Can you work these out from the model? Positions are in its coordinate system, mm. Face numbers are marked on the shaded views. A direction names the side the tool comes from. Give positions to 0.01 mm unless a question says otherwise; leave off trailing zeros. Write each loop counter-clockwise with the first axis right and the second up, starting at its lowest first coordinate (ties: lowest second). Pieces come first, ordered by that corner, then holes.
Autodesk Inventor part; units mm, degrees
ref_plane "YZ Plane" through (0, 0, 0) normal (1, 0, 0) x (0, 1, 0)
ref_plane "XZ Plane" through (0, 0, 0) normal (0, 1, 0) x (-1, 0, 0)
ref_plane "XY Plane" through (0, 0, 0) normal (0, 0, 1) x (1, 0, 0)
sketch "スケッチ1" plane through (0, 0, 0) normal (0, 0, 1) x (1, 0, 0)
  circle A0 centre (0, 0) radius 46.9412
  dimension "d3" = 93.8824
extrude "押し出し1" add sketch "スケッチ1" along normal blind 10.5
sketch "スケッチ2" plane through (0, 0, 10.5) normal (0, 0, 1) x (1, 0, 0)
  circle A0 centre (0, 0) radius 46.9412
  arc A1 (35.7361, 3.8892) -> (3.8892, 35.7361) centre (0, 0) ccw
  circle A2 centre (29.2617, 29.2617) radius 2.1
  circle A3 centre (-39.9723, 10.7105) radius 2.1
  circle A4 centre (10.7105, -39.9723) radius 2.1
  circle A5 centre (0, 0) radius 35.9471
  dimension "d4" = 4.2
extrude "押し出し2" cut sketch "スケッチ2" against normal blind 5 contours A5 A1
sketch "スケッチ3" plane through (0, 0, 10.5) normal (0, 0, 1) x (1, 0, 0)
  circle A0 centre (0, 0) radius 46.9412
  arc A1 (-5.0225, 35.5945) -> (35.5945, -5.0225) centre (0, 0) ccw
  arc A2 (35.7361, 3.8892) -> (3.8892, 35.7361) centre (0, 0) ccw
  circle A3 centre (29.2617, 29.2617) radius 2.1
  circle A4 centre (-39.9723, 10.7105) radius 2.1
  circle A5 centre (10.7105, -39.9723) radius 2.1
  circle A6 centre (0, 0) radius 35.9471
  dimension "d7" = 4.2
extrude "押し出し3" cut sketch "スケッチ3" against normal blind 10.5 contours A3 | A4 | A5
sketch "スケッチ4" plane through (0, 0, 5.5) normal (0, 0, 1) x (1, 0, 0)
  circle A0 centre (0, 0) radius 10.5
  circle A1 centre (0, 0) radius 10.5
extrude "押し出し4" cut sketch "スケッチ4" against normal blind 10.5
sketch "スケッチ5" plane through (0, 0, 5.5) normal (0, 0, 1) x (1, 0, 0)
  circle A0 centre (0, 0) radius 10.5
  circle A1 centre (0, 0) radius 35.9471
  circle A2 centre (0, 0) radius 13.5
  circle A3 centre (0, 0) radius 32.9471
  dimension "d12" = 3
  dimension "d13" = 3
extrude "押し出し5" cut sketch "スケッチ5" against normal blind 2 contours A3
sketch "スケッチ6" plane through (0, 0, 5.5) normal (0, 0, 1) x (1, 0, 0)
  point P0 (0, 0)
sketch "スケッチ7" plane through (0, 0, 5.5) normal (0, 0, 1) x (1, 0, 0)
  circle A0 centre (0, 0) radius 38.9471
  circle A1 centre (0, 0) radius 35.9471
  dimension "d16" = 3
extrude "押し出し6" cut sketch "スケッチ7" along normal blind 2.5
properties part number "fix_plate_2"
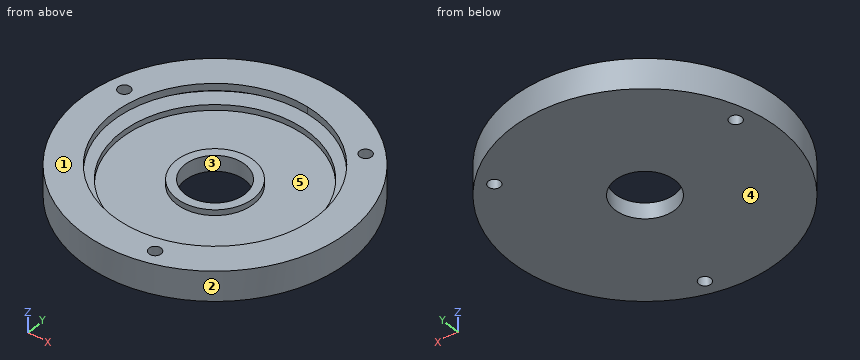
(1) Imagine slicing it at C-C, the plane z = 2. Write out the boundary of the cut face in (x, y), plus the area to 3 significant figures.
Returned:
outline: circle Ø93.88 at (0, 0); hole circle Ø4.2 at (-39.97, 10.71); hole circle Ø21 at (0, 0); hole circle Ø4.2 at (10.71, -39.97); hole circle Ø4.2 at (29.26, 29.26)
area: 6,530 mm2
(2) Imagine slicing it at D-D, the plane y = 22.5. Write out the boundary of the cut face in (x, z).
Returned:
outline: (-41.2, 0) - (41.2, 0) - (41.2, 10.5) - (28.03, 10.5) - (28.03, 8) - (31.79, 8) - (31.79, 5.5) - (24.07, 5.5) - (24.07, 3.5) - (-24.07, 3.5) - (-24.07, 5.5) - (-31.79, 5.5) - (-31.79, 8) - (-28.03, 8) - (-28.03, 10.5) - (-41.2, 10.5) - close
(3) Imagine slicing it at B-B, the plane x = 1. Write out the boundary of the cut face in (y, z).
Returned:
outline: (-46.93, 0) - (-10.45, 0) - (-10.45, 5.5) - (-13.46, 5.5) - (-13.46, 3.5) - (-32.93, 3.5) - (-32.93, 5.5) - (-38.93, 5.5) - (-38.93, 8) - (-35.93, 8) - (-35.93, 10.5) - (-46.93, 10.5) - close; (10.45, 0) - (46.93, 0) - (46.93, 10.5) - (35.93, 10.5) - (35.93, 8) - (38.93, 8) - (38.93, 5.5) - (32.93, 5.5) - (32.93, 3.5) - (13.46, 3.5) - (13.46, 5.5) - (10.45, 5.5) - close
(4) Will these pins go through, and if not, where does the flat tip stop? P1, Ø23.5, axis at x = 2.5, y = -13, coming from the -Z side; P2, Ø5, axis at x = -27, y = -1, coming from the +Z side; P3, Ø4, axis at x = -12.5, z = 4, coming from the -Y side; P4, Ø13.5, axis at x = 6.5, y = -1, coming from the +Z side.
Returned:
P1: stops at z = 0
P2: stops at z = 3.5
P3: stops at y = -45.75
P4: stops at z = 5.5
(5) If I drill on L1, parallel to Y at x = 0, z = 4.45; L2, parallel to X at y = -11.5, z = 4.75; L3, parallel to Z at x = -10.5, y = -35, over which ranges is the centre line in solid material (lowest first)?
Returned:
L1: y = -46.94 to -32.95, -13.5 to -10.5, 10.5 to 13.5, 32.95 to 46.94
L2: x = -45.51 to -30.87, -7.07 to 7.07, 30.87 to 45.51
L3: z = 0 to 5.5, 8 to 10.5
(6) Imagine slicing it at A-A, the plane y = 0. Write out the boundary of the cut face in (x, z), plus the area to 3 significant figures.
Returned:
outline: (-46.94, 0) - (-10.5, 0) - (-10.5, 5.5) - (-13.5, 5.5) - (-13.5, 3.5) - (-32.95, 3.5) - (-32.95, 5.5) - (-38.95, 5.5) - (-38.95, 8) - (-35.95, 8) - (-35.95, 10.5) - (-46.94, 10.5) - close; (10.5, 0) - (46.94, 0) - (46.94, 10.5) - (35.95, 10.5) - (35.95, 8) - (38.95, 8) - (38.95, 5.5) - (32.95, 5.5) - (32.95, 3.5) - (13.5, 3.5) - (13.5, 5.5) - (10.5, 5.5) - close
area: 418 mm2
(7) If we mould it in two halves opening along X, with no side actions, what happens to the marked faces 1, 2 and 3? For each: +X half, -X half, draft (parallel to the pull), parting line (faces both ways), or undercut.
Returned:
face 1: draft
face 2: parting line
face 3: undercut
(8) For the marked faces 4 and 5, which set-ups out of +Z, -Z, +X, -X, +Y, -Y let a thin tool reach every point of the face, with its end or its side?
Returned:
face 4: -Z, +X, -X, +Y, -Y
face 5: +Z
